Read the model definition and answer for the solid it produces. Units are mm, in the model's axes. A direction names the side the tool comes from. Coordinates: 2 decimals unless noted, no trailing zeros. Order: outer loops, then holes, each group sorted by start corner. A loop starts at its lowest first (then second) coordinate and runs counter-clockwise, first axis right, second up. Notation, with made-up numbers: (80.25, 33.5) - (92.25, 33.5) arc R32 ccw to (92.25, 69.5) - close; hole circle Ø11 at (86.5, 41.5). An arc over 180 degrees is marked (long way). Use one line per item in the form item = value.
```python
from build123d import *

# Parameters (mm, degrees)
BOSS_EXTRUDE1_DEPTH = 19.5
SKETCH5_W           = 6.000098135
SKETCH5_H           = 3
BOSS_EXTRUDE2_DEPTH = 40
FILLET1_R           = 2
SKETCH6_R           = 1.5
CUT_EXTRUDE1_DEPTH  = 4


with BuildPart() as part:
    # Sketch3 → Boss-Extrude1 (new body)
    with BuildSketch(Plane.XZ.offset(9.5)):
        Polygon((20.540895742, -1), (26.540993877, -1), (26.523835555, 2), (20.52373742, 2), align=None)
    extrude(amount=-BOSS_EXTRUDE1_DEPTH)

    # Sketch5 → Boss-Extrude2 (add)
    with BuildSketch(Plane.XY.offset(2)):
        with Locations((23.523786488, 8.5)):
            Rectangle(SKETCH5_W, SKETCH5_H)
    extrude(amount=BOSS_EXTRUDE2_DEPTH)

    # Fillet1
    fillet1_edges = [part.edges().sort_by_distance(p)[0] for p in [
        (23.540944809, 10, -1),
    ]]
    fillet(fillet1_edges, radius=FILLET1_R)

    # Sketch6 → Cut-Extrude1 (cut, through all)
    with BuildSketch(Plane.XZ.offset(-7)):
        with Locations((23.5, 38)):
            Circle(SKETCH6_R)
        with Locations((23.5, 29)):
            Circle(SKETCH6_R)
    extrude(amount=-CUT_EXTRUDE1_DEPTH, mode=Mode.SUBTRACT)


solid = part.part
```
(1) Section B-B, the plane z = 29 is taken. Write down the section's boundary in (x, y), then the cut area to 3 significant figures.
Answer list:
outline = (20.52, 7) - (22, 7) - (22, 10) - (20.52, 10) - close; (25, 7) - (26.52, 7) - (26.52, 10) - (25, 10) - close
area = 9.00 mm2
(2) Section D-D, the plane y = -6.5 is taken. Write down the section's boundary in (x, z).
Answer list:
outline = (20.52, 2) - (20.54, -1) - (26.54, -1) - (26.52, 2) - close
(3) Straight lines are drawn through the part: L1, parallel to Z at x = 23.5, y = 9.35; L2, parallel to Y at x = 25.5, z = 39; L3, parallel to Z at x = 23.5, y = -8.25. For each, find the intervals that lie inside material, in ascending order.
Answer list:
L1 = -0.48 to 27.5, 30.5 to 36.5, 39.5 to 42
L2 = 7 to 10
L3 = -1 to 2
(4) Given pin 1 Ø3 at (x, z) = (24.5, 17) entering from -Y; pin 2 Ø1.5 at (x, y) = (25.5, -5) entering from +Z; pin 3 Ø1.5 at (y, z) = (8.5, 27) entering from +X, each flat-ended and moving along its own axis, determine where each tip first touches the part or whether it passes through.
Answer list:
pin_1 = 7
pin_2 = 2
pin_3 = 26.52
(5) Which of the six approach directions +Z, -Z, +X, -X, +Y, -Y give full straight-line access (tool end or side, diameter ignored) to faces 4 (the flat face through (23, -1, -1)), 5 (the flat face through (23, 7, 22))?
Answer list:
face_4 = -Z, +X, -X, +Y, -Y
face_5 = +Z, +X, -X, -Y
(6) The mould has two halves that part along X. Classify faces 1 (the flat face through (20.524, 8, 22)), 2 (the flat face through (24, -1, 2)), 3 (the cylindrical face through (23.175, 8.479, 36.536)): +X half, -X half, draft (parallel to the pull), parting line (faces both ways), or undercut.
Answer list:
face_1 = -X half
face_2 = draft
face_3 = undercut
(7) Section C-C, the plane x = 25.75 is taken. Write down the section's boundary in (y, z).
Answer list:
outline = (-9.5, -1) - (8, -1) arc R2 ccw to (10, 1) - (10, 42) - (7, 42) - (7, 2) - (-9.5, 2) - close
(8) Section A-A, the plane x = 23.5 is taken. Write down the section's boundary in (y, z).
Answer list:
outline = (-9.5, -1) - (8, -1) arc R2 ccw to (10, 1) - (10, 27.5) - (7, 27.5) - (7, 2) - (-9.5, 2) - close; (7, 30.5) - (10, 30.5) - (10, 36.5) - (7, 36.5) - close; (7, 39.5) - (10, 39.5) - (10, 42) - (7, 42) - close
